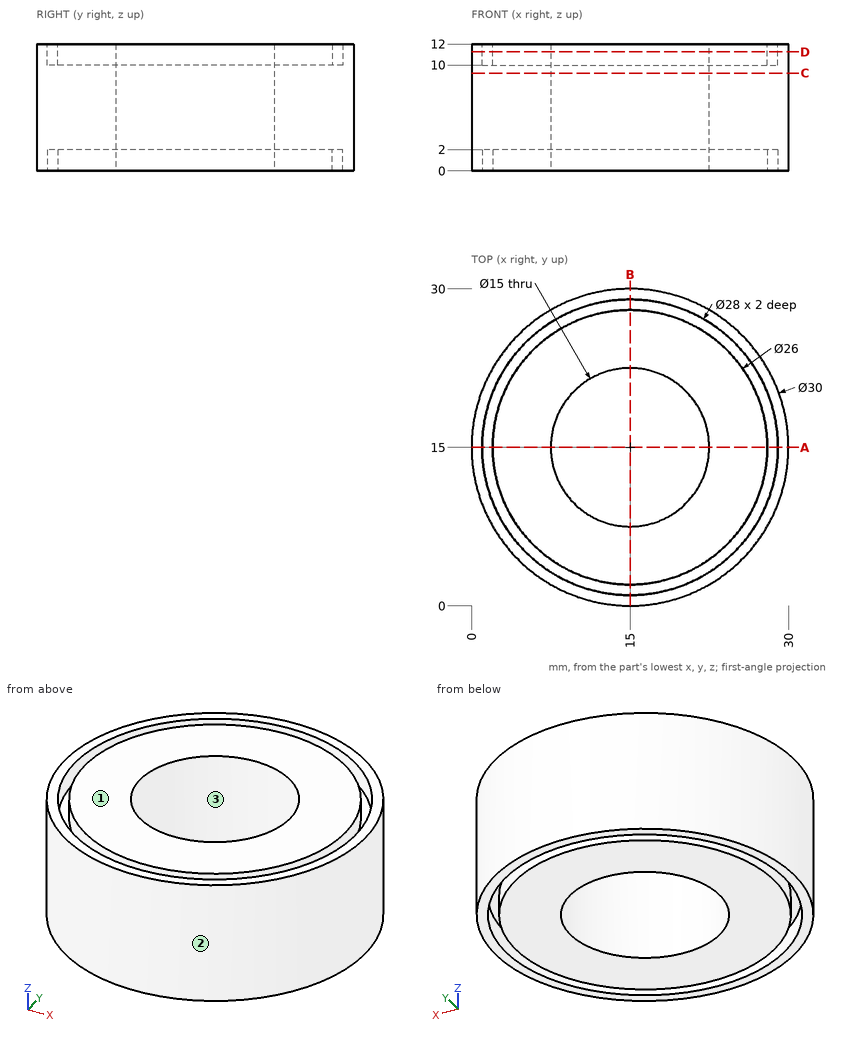
Geometry: see drawing. Coordinates: mm, zero at the bounding-box minimum. Coordinates: 2 decimals unless noted, no trailing zeros. Loops run counter-clockwise (first coordinate to the right, second up) from the corner with the lowest first, then second, coordinate; pieces in that order, holes last. Notation, with made-up numbers: M 8.5,60 L 55.5,60 A14 ccw 55.5,81 Z; hole C 28,39 d9. An arc over 180 degrees is marked long. Put each result on its own line as item: value. Start each with the question number.
1) Cut plane D-D on z = 11.25. Return the cut outline in (x, y).
2) Cut plane C-C on z = 9.25. Return the cut outline in (x, y).
3) Contact query for flat-ended pins moving along their axis: pin 1 Ø3 at (x, z) = (26.5, 4.5) entering from +Y; pin 2 Ø5 at (x, z) = (4, 7.5) entering from -Y; pin 3 Ø5 at (y, z) = (25, 6.5) entering from +X. Output: stop coordinate, or through.
4) Ray query, L1, parallel to Y at x = 15, z = 11.3; L2, parallel to Y at x = 20, z = 1.5; L3, parallel to Y at x = 15, z = 6. Return the intervals inside material, ascending. Write a range as from..to.
5) Cut plane A-A on y = 15. Return the cut outline in (x, z), then the cut area to 3 significant figures.
6) Pull-direction query (X, two-part tool) for the marked faces 1, 2 and 3; classes: pulls with the +X half, pulls with the -X half, needs draft (parallel to the pull), parting line crosses it, or undercut.
The answers:
1. outline: C 15,15 d30; C 15,15 d26; hole C 15,15 d28; hole C 15,15 d15
2. outline: C 15,15 d30; hole C 15,15 d15
3. pin 1: stops at y = 26.18
3. pin 2: stops at y = 2.64
3. pin 3: stops at x = 27.99
4. L1: y = 0..1, 2..7.5, 22.5..28, 29..30
4. L2: y = 0.86..1.92, 3..9.41, 20.59..27, 28.08..29.14
4. L3: y = 0..7.5, 22.5..30
5. outline: M 0,0 L 1,0 L 1,2 L 2,2 L 2,0 L 7.5,0 L 7.5,12 L 2,12 L 2,10 L 1,10 L 1,12 L 0,12 Z; M 22.5,0 L 28,0 L 28,2 L 29,2 L 29,0 L 30,0 L 30,12 L 29,12 L 29,10 L 28,10 L 28,12 L 22.5,12 Z
5. area: 172 mm²
6. face 1: needs draft
6. face 2: parting line crosses it
6. face 3: undercut
